The drawing under review shows one solid part. Ordinate dimensions are in mm from its lowest x, y, z. Give positions to 0.01 mm unless a question says otherwise; leave off trailing zeros. Order: outer loops, then holes, each group sorted by start corner. A loop starts at its lowest first (then second) coordinate and runs counter-clockwise, first axis right, second up. Notation, with made-up numbers: (-20.5, 61.5) - (7.5, 61.5) arc R23 cw to (7.5, 72.5) - close; hole circle Ø4 at (68, 25). An arc over 180 degrees is marked (long way). Use CSV: the item, a comma, the result in double quotes.
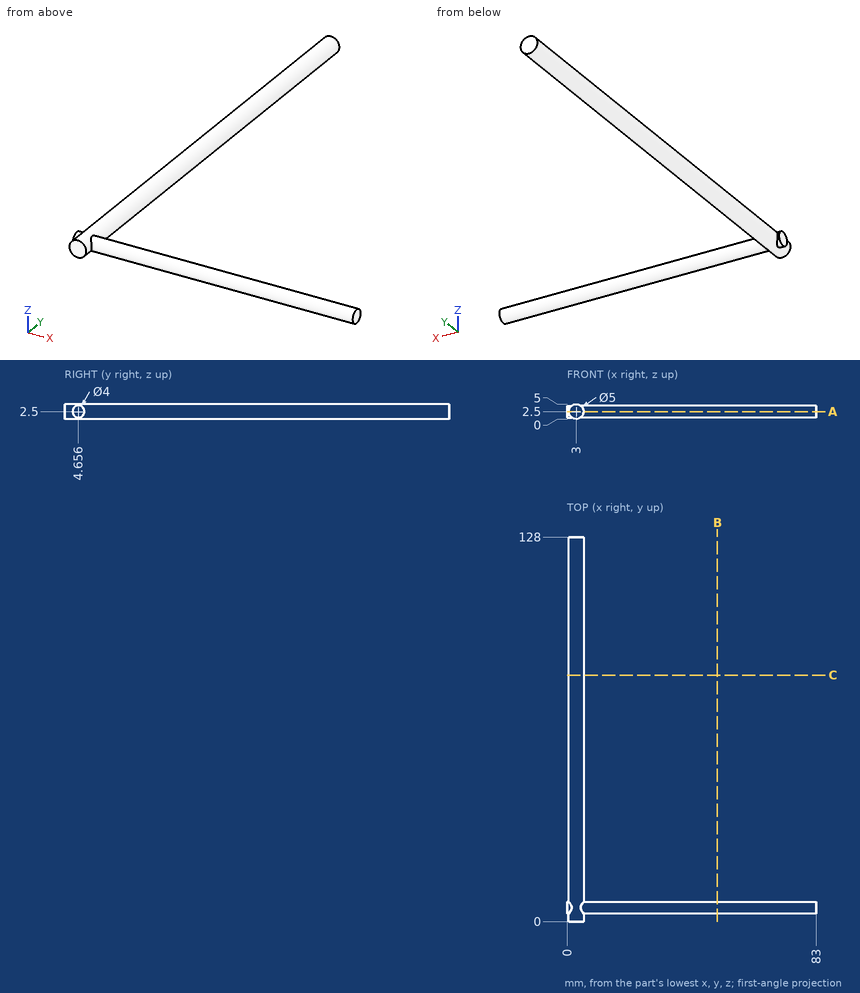
Item 1: Take a section at A-A, the plane z = 2.5. Give the boundary of the cut face in (x, y).
Results list:
outline,"(0, 2.66) - (0.5, 2.66) - (0.5, 0) - (5.5, 0) - (5.5, 2.66) - (83, 2.66) - (83, 6.66) - (5.5, 6.66) - (5.5, 128) - (0.5, 128) - (0.5, 6.66) - (0, 6.66) - close"
Item 2: Clearance check with flat-ended pins moving along their axes: pin 1 (2 mm diameter, centred on x = 37, z = 3.5, fed in from -Y); pin 2 (10 mm diameter, centred on x = 11.5, y = 17.5, fed in from +Z). State where each tip first meets the part, or that it passes through.
Results list:
pin 1,"stops at y = 2.66"
pin 2,"passes through"
Item 3: Take a section at C-C, the plane y = 82. Give the boundary of the cut face in (x, z).
Results list:
outline,"circle Ø5 at (3, 2.5)"
Item 4: Take a section at B-B, the plane x = 50. Give the boundary of the cut face in (y, z), and give its area (3 significant figures).
Results list:
outline,"circle Ø4 at (4.66, 2.5)"
area,"12.6 mm2"
Item 5: Wall thickness on L1, parallel to X at y = 40.5, z = 2.7; L2, parallel to X at y = 120, z = 4.5; L3, parallel to Y at x = 63, z = 2.6: over which ranges is each line inside the solid? List them lowest first.
Results list:
L1,"x = 0.51 to 5.49"
L2,"x = 1.5 to 4.5"
L3,"y = 2.66 to 6.65"
